The figure shows three views and two pictorial views of one solid part (mm, origin at its lowest corner). Answer the questions. Give positions to 0.01 mm unless a question says otherwise; leave off trailing zeros. Loops run counter-clockwise (first coordinate to the right, second up) from the corner with the lowest first, then second, coordinate; pieces in that order, holes last. Notation, with made-up numbers: (-11, 53) - (-5, 53) arc R23 cw to (-5, 68) - close; hole circle Ø7 at (14.25, 74). An arc over 180 degrees is marked (long way). Use a Markdown table: item, result. Add a question column.
Item 1: Consider probe 1 along X at (y, z) = (11.25, 30); probe 2 along X at (y, z) = (1.25, 35). Determine where each line is inside the solid, lowest interval first. Write a range as [from, to].
Item 2: A cutting plane is placed at A-A (y = 5.5). Determine the outline of the cut face in (x, z).
Item 3: Each of these flat-tipped pins is pushed along its axis until it touches: P1, Ø4, axis at y = 4, z = 38, coming from the +X side; P2, Ø3, axis at y = 13.5, z = 21.5, coming from the -X side; P3, Ø6, axis at y = 4.5, z = 34, coming from the -X side. Where does it stop, or does it pass through?
Item 4: A cutting plane is placed at B-B (z = 77). Determine the outline of the cut face in (x, y), plus the area to 3 significant figures.
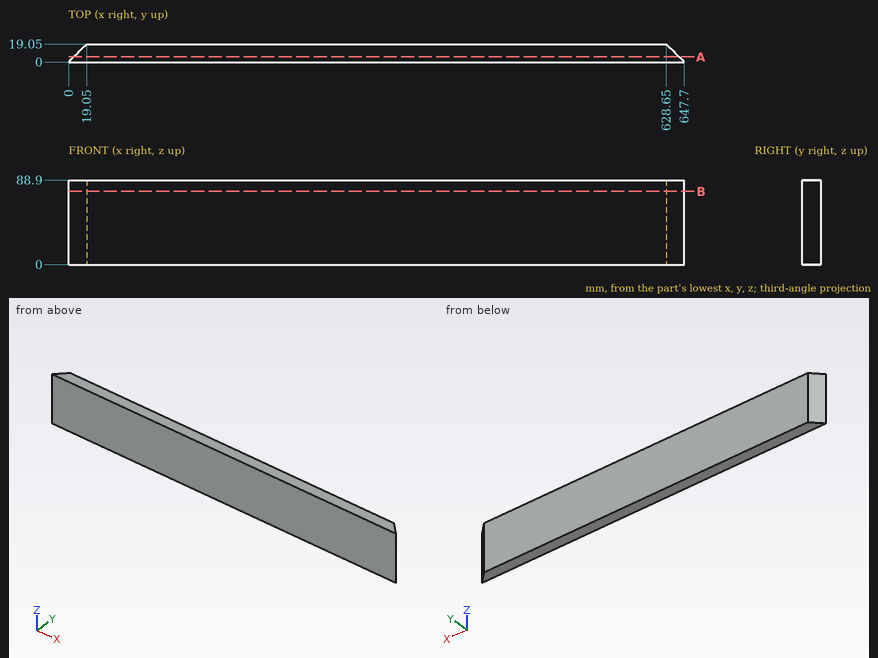
Geometry says:
| question | item | result |
|---|---|---|
| 1 | probe 1 | [11.25, 636.45] |
| 1 | probe 2 | [1.25, 646.45] |
| 2 | outline | (5.5, 0) - (642.2, 0) - (642.2, 88.9) - (5.5, 88.9) - close |
| 3 | P1 | x = 645.7 |
| 3 | P2 | x = 12 |
| 3 | P3 | x = 1.5 |
| 4 | outline | (0, 0) - (647.7, 0) - (628.65, 19.05) - (19.05, 19.05) - close |
| 4 | area | 12,000 mm² |
